Design review of the part built by this model. Coordinates are the model's own, in mm. A direction names the side the tool comes from. Round coordinates to 2 decimals unless told otherwise and drop trailing zeros. Loops run counter-clockwise (first coordinate to the right, second up) from the corner with the lowest first, then second, coordinate; pieces in that order, holes last. Notation, with made-up numbers: (29.25, 81.5) -> (40.25, 81.5) arc R22 cw to (40.25, 101.5) -> close; hole circle Ø8 at (-8, 78.5). An arc over 180 degrees is marked (long way). Use a Markdown table: item, result. Add a question column.
from build123d import *

# Parameters (mm, degrees)
CROQUIS1_R              = 33
CROQUIS1_R_2            = 17.5
SALIENTE_EXTRUIR1_DEPTH = 19
REDONDEO1_R             = 2
REDONDEO2_R             = 2


with BuildPart() as part:
    # Croquis1 → Saliente-Extruir1 (new body, symmetric)
    with BuildSketch(Plane.XY):
        Circle(CROQUIS1_R)
        Circle(CROQUIS1_R_2, mode=Mode.SUBTRACT)
    extrude(amount=SALIENTE_EXTRUIR1_DEPTH, both=True)

    # Croquis2 → Cortar-Revolución1 (revolve, cut)
    with BuildSketch(Plane(origin=(0, 0, 0), x_dir=(1, 0, 0), z_dir=(0, 1, 0))):
        with BuildLine():
            Line((17.75, 0.5), (18.5, 0.5))
            Line((18.5, 0.5), (18.5, -0.5))
            Line((18.5, -0.5), (17.75, -0.5))
            ThreePointArc((17.75, -0.5), (17.573223305, -0.426776695), (17.5, -0.25))
            Line((17.5, -0.25), (17.5, 0.25))
            ThreePointArc((17.5, 0.25), (17.573223305, 0.426776695), (17.75, 0.5))
        make_face()
    revolve(axis=Axis((0, 0, 0), (0, 0, -1)), mode=Mode.SUBTRACT)

    # Redondeo1
    redondeo1_edges = [part.edges().sort_by_distance(p)[0] for p in [
        (-17.5, 0, 19),
    ]]
    fillet(redondeo1_edges, radius=REDONDEO1_R)

    # Croquis3 → Cortar-Revolución2 (revolve, cut)
    with BuildSketch(Plane(origin=(0, 0, 0), x_dir=(0, 0, -1), z_dir=(1, 0, 0))):
        Polygon((-19, 23.5), (-19, 31.5), (-18, 31.5), (-18, 30), (-18.2, 30), (-18.2, 27.5), (-18.3, 27.5), (-18.3, 23.5), align=None)
    cortar_revoluci_n2 = revolve(axis=Axis((0, 0, 0), (0, 0, 1)), mode=Mode.SUBTRACT)

    # Redondeo2
    redondeo2_edges = [part.edges().sort_by_distance(p)[0] for p in [
        (-17.5, 0, -19),
    ]]
    fillet(redondeo2_edges, radius=REDONDEO2_R)

    # Simetría1: Cortar-Revolución2 across plane
    add(cortar_revoluci_n2.mirror(Plane.XY), mode=Mode.SUBTRACT)


solid = part.part
1. To check wall thickness, follow probe 1 along Y at (x, z) = (0, -18.75); probe 2 along Y at (x, z) = (0, 18.25); probe 3 along Z at (x, y) = (25.5, 3.5). State the ranges of each line that lie inside material, in increasing order. Write a range as from..to.
2. Consider section B-B on y = 26. State the section outline as (x, z) points, plus the area to 3 significant figures.
3. Mouldability with a two-part tool opening along Y and no side actions: class faces 1 (the face through (-4.01, 18.06, 0.01)), 2 (the face through (16.53, -6.94, -0.5)), 3 (the face through (30.5, -12.6, 0.3)), 4 (the face through (-9, 18, 19)) as +Y half, -Y half, draft (parallel to the pull), parting line (faces both ways), or undercut.
4. Insertion check: P1, Ø10, axis at x = 11.5, z = -5.5, coming from the -Y side; P2, Ø3, axis at y = 8.5, z = -5.5, coming from the -X side; P3, Ø4, axis at x = 9.5, y = -25.5, coming from the +Z side. Each pin has a flat end and moves straight along its axis. Give the tip position at first contact, or say it passes through.
5. For faces 5 (the face through (-13.887, -10.648, 8.508)), 6 (the face through (-7.1, 22.4, 18.7)), 7 (the face through (-7.1, 22.4, -18.7)), list the 3-axis set-ups (+Z, -Z, +X, -X, +Y, -Y) from which the entire face can be reached by the end or side of a thin tool; tool diameter is ignored.
6. Consider section C-C on x = -25.5. State the section outline as (y, z) points, plus the area to 3 significant figures.
7. Consider section A-A on z = -9. State the section outline as (x, y) points.
Verdict:
| question | item | result |
|---|---|---|
| 1 | probe 1 | y = -33..-31.5, -23.5..-18.53, 18.53..23.5, 31.5..33 |
| 1 | probe 2 | y = -33..-31.5, -27.5..-17.94, 17.94..27.5, 31.5..33 |
| 1 | probe 3 | z = -18.3..18.3 |
| 2 | outline | (-20.32, -19) -> (-17.78, -19) -> (-17.78, -18) -> (-14.97, -18) -> (-14.97, -18.2) -> (-8.96, -18.2) -> (-8.96, -18.3) -> (8.96, -18.3) -> (8.96, -18.2) -> (14.97, -18.2) -> (14.97, -18) -> (17.78, -18) -> (17.78, -19) -> (20.32, -19) -> (20.32, 19) -> (17.78, 19) -> (17.78, 18) -> (14.97, 18) -> (14.97, 18.2) -> (8.96, 18.2) -> (8.96, 18.3) -> (-8.96, 18.3) -> (-8.96, 18.2) -> (-14.97, 18.2) -> (-14.97, 18) -> (-17.78, 18) -> (-17.78, 19) -> (-20.32, 19) -> close |
| 2 | area | 1,490 mm² |
| 3 | face 1 | undercut |
| 3 | face 2 | undercut |
| 3 | face 3 | parting line |
| 3 | face 4 | draft |
| 4 | P1 | stops at y = -32.35 |
| 4 | P2 | stops at x = -32.25 |
| 4 | P3 | stops at z = 18.3 |
| 5 | face 5 | +Z, -Z |
| 5 | face 6 | +Z |
| 5 | face 7 | -Z |
| 6 | outline | (-20.95, -19) -> (-18.49, -19) -> (-18.49, -18) -> (-15.8, -18) -> (-15.8, -18.2) -> (-10.3, -18.2) -> (-10.3, -18.3) -> (10.3, -18.3) -> (10.3, -18.2) -> (15.8, -18.2) -> (15.8, -18) -> (18.49, -18) -> (18.49, -19) -> (20.95, -19) -> (20.95, 19) -> (18.49, 19) -> (18.49, 18) -> (15.8, 18) -> (15.8, 18.2) -> (10.3, 18.2) -> (10.3, 18.3) -> (-10.3, 18.3) -> (-10.3, 18.2) -> (-15.8, 18.2) -> (-15.8, 18) -> (-18.49, 18) -> (-18.49, 19) -> (-20.95, 19) -> close |
| 6 | area | 1,530 mm² |
| 7 | outline | circle Ø66 at (0, 0); hole circle Ø35 at (0, 0) |
